For this review, take the finished solid that the model builds, in its own axes (mm). A direction names the side the tool comes from. Coordinates: 2 decimals unless noted, no trailing zeros. Loops run counter-clockwise (first coordinate to the right, second up) from the corner with the lowest first, then second, coordinate; pieces in that order, holes last. Notation, with made-up numbers: (23, 71) -> (59, 71) arc R28 ccw to (59, 95) -> close; hole circle Ø10 at (41, -21). An arc over 180 degrees is marked (long way). Answer in a Markdown table with one row per item.
Autodesk Inventor part; units mm, degrees
ref_plane "YZ Plane" through (0, 0, 0) normal (1, 0, 0) x (0, 1, 0)
ref_plane "XZ Plane" through (0, 0, 0) normal (0, 1, 0) x (-1, 0, 0)
ref_plane "XY Plane" through (0, 0, 0) normal (0, 0, 1) x (1, 0, 0)
sketch "Эскиз1" plane through (0, 0, 0) normal (0, 1, 0) x (-1, 0, 0)
  line L0 (0, 0) -> (30, 0)
  line L1 (30, 0) -> (30, -1.5)
  line L2 (30, -1.5) -> (0, -1.5)
  line L3 (0, -1.5) -> (0, 0)
  line L4 (0, -1.5) -> (1.5, -1.5)
  line L5 (1.5, -1.5) -> (1.5, -25)
  line L6 (1.5, -25) -> (0, -25)
  line L7 (0, -25) -> (0, -1.5)
  dimension "d0" = 1.5
  dimension "d1" = 25
  dimension "d2" = 30
  dimension "d3" = 1.5
extrude "Выдавливание1" add sketch "Эскиз1" along normal mid plane 27
sketch "Эскиз2" plane through (-1.5, -13.5, -1.5) normal (0, 0, -1) x (-1, 0, 0)
  line L0 (28.5, 27) -> (-1.5, 27) construction
  line L1 (23.581, 27) -> (23.581, 0.3508) construction
  line L2 (28.5, 0) -> (28.5, 27) construction
  line L3 (28.5, 13.5) -> (-1.5, 13.5) construction
  circle A0 centre (23.581, 21) radius 1.5
  circle A1 centre (23.581, 6) radius 1.5
  line L4 (0, 0) -> (0, 27)
  line L5 (0, 17.5) -> (15.5309, 17.5)
  line L6 (15.5309, 17.5) -> (15.5309, 9.5)
  line L7 (15.5309, 9.5) -> (0, 9.5)
  line L8 (0, 9.5) -> (0, 17.5)
  line L9 (28.5, 0) -> (0, 0)
  dimension "d6" = 3
  dimension "d7" = 3
  dimension "d8" = 15
  dimension "d9" = 7.5
  dimension "d10" = 9.5
  dimension "d11" = 15.5309
  dimension "d12" = 9.5
extrude "Выдавливание2" cut sketch "Эскиз2" against normal blind 27 contours L4 L5 L6 L7
fillet "Сопряжение1" radius 1 2 edges at (-1.5, 8.75, -1.5) (-1.5, -8.75, -1.5)
fillet "Сопряжение2" radius 3 1 edges at (0, 0, 0)
extrude "Выдавливание3" cut sketch "Эскиз2" against normal blind 27 contours A0 | A1
sketch "Эскиз3" plane through (-1.5, -13.5, -25) normal (-1, 0, 0) x (0, 0, 1)
  circle A0 centre (3.2567, 9.1412) radius 1.5
  circle A1 centre (11.2567, 23.1412) radius 1.5
  point P0 (25, 13.5)
  dimension "d19" = 3
  dimension "d20" = 3
  dimension "d23" = 14
  dimension "d24" = 8
extrude "Выдавливание4" cut sketch "Эскиз3" against normal blind 27
fillet "Сопряжение3" radius 5 2 edges at (-30, -13.5, -0.75) (-30, 13.5, -0.75)
fillet "Сопряжение4" radius 2 2 edges at (-0.75, -13.5, -25) (-0.75, 13.5, -25)
properties part number "крепление концевика"
Item 1: Take a section at A-A, the plane y = -1.25. State the section outline as (x, z) points, and give its area (3 significant figures).
Worked answers:
| item | result |
|---|---|
| outline | (-30, -1.5) -> (-17.03, -1.5) -> (-17.03, 0) -> (-30, 0) -> close; (-1.5, -25) -> (0, -25) -> (0, -3) arc R3 ccw to (-1.5, -0.4) -> close |
| area | 55.2 mm² |
Item 2: Take a section at C-C, the plane y = 4.5. State the section outline as (x, z) points, and give its area (3 significant figures).
Worked answers:
| item | result |
|---|---|
| outline | (-30, -1.5) -> (-2.5, -1.5) arc R1 cw to (-1.5, -2.5) -> (-1.5, -25) -> (0, -25) -> (0, -3) arc R3 ccw to (-3, 0) -> (-30, 0) -> close |
| area | 78.5 mm² |
Item 3: For faces 4 (the flat face through (-9, -4, -1)), 5 (the flat face through (-19, 0, -1.5)), 6 (the flat face through (-30, 0, -1)), list the 3-axis set-ups (+Z, -Z, +X, -X, +Y, -Y) from which the entire face can be reached by the end or side of a thin tool; tool diameter is ignored.
Worked answers:
| item | result |
|---|---|
| face 4 | +Z, -Z |
| face 5 | -Z, -X, +Y, -Y |
| face 6 | +Z, -Z, -X, +Y, -Y |
Item 4: The part is to be moulded in two halves that separate along X. For faces 1 (the cylindrical face through (-26.47, -8.07, -0.76)), 2 (the flat face through (0, 0, -14)), 3 (the cylindrical face through (-0.76, 10.655, -14.849)), say which applies: +X half, -X half, draft (parallel to the pull), parting line (faces both ways), or undercut.
Worked answers:
| item | result |
|---|---|
| face 1 | undercut |
| face 2 | +X half |
| face 3 | draft |
Item 5: Take a section at D-D, the plane y = 7.5. State the section outline as (x, z) points.
Worked answers:
| item | result |
|---|---|
| outline | (-30, -1.5) -> (-26.58, -1.5) -> (-26.58, 0) -> (-30, 0) -> close; (-23.58, -1.5) -> (-2.5, -1.5) arc R1 cw to (-1.5, -2.5) -> (-1.5, -25) -> (0, -25) -> (0, -3) arc R3 ccw to (-3, 0) -> (-23.58, 0) -> close |
Item 6: Insertion check: pin 1 (4 mm diameter, centred on x = -24, y = -2, fed in from -Z); pin 2 (1.5 mm diameter, centred on y = -8.5, z = -9, fed in from -X); pin 3 (0.8 mm diameter, centred on y = 0.5, z = -1, fed in from +X). Each pin has a flat end and moves straight along its axis. Give the tip position at first contact, or say it passes through.
Worked answers:
| item | result |
|---|---|
| pin 1 | z = -1.5 |
| pin 2 | x = -1.5 |
| pin 3 | x = -0.46 |
Item 7: For L1, parallel to Y at x = -26.25, z = -1; L2, parallel to X at y = 11, z = -9.25, list the stretches that pass through material, from the lowest coordinate up.
Worked answers:
| item | result |
|---|---|
| L1 | -13.34 to -8.44, -6.56 to 6.56, 8.44 to 13.34 |
| L2 | -1.5 to 0 |
Item 8: Take a section at B-B, the plane x = -7.5. State the section outline as (y, z) points.
Worked answers:
| item | result |
|---|---|
| outline | (-13.5, -1.5) -> (-4, -1.5) -> (-4, 0) -> (-13.5, 0) -> close; (4, -1.5) -> (13.5, -1.5) -> (13.5, 0) -> (4, 0) -> close |
